Source: three-view drawing plus pictorial views. Frame: mm from the lowest corner of the part. Round coordinates to 2 decimals unless told otherwise and drop trailing zeros. Order: outer loops, then holes, each group sorted by start corner. A loop starts at its lowest first (then second) coordinate and runs counter-clockwise, first axis right, second up. Notation, with made-up numbers: (4, 81.25) -> (58, 81.25) arc R14 cw to (58, 100.25) -> close; hole circle Ø6 at (64.25, 50.25). An arc over 180 degrees is marked (long way). Answer as CSV lines item,"result". Start each with the question number.
1) Section query B-B, the plane y = 10.25. Output: boundary loops of the cut face in (x, z) (3 decimals), and give its area (3 significant figures).
2) Section query D-D, the plane z = 177.5. Output: boundary loops of the cut face in (x, y).
3) Section query A-A, the plane x = 150. Output: boundary loops of the cut face in (y, z), and give its area (3 significant figures).
4) First-contact query: P1, Ø10, axis at x = 40.5, y = 7, coming from the -Z side; P2, Ø5.5, axis at y = 5.5, z = 276, coming from the -X side; P3, Ø4, axis at y = 10.5, z = 310.5, coming from the +X side. Flat tips, straight axial feed; report the tip coordinate or a pass-through.
5) Section query C-C, the plane z = 68.5. Output: boundary loops of the cut face in (x, y).
6) Line query: L1, parallel to X at y = 4.25, z = 31.5; L2, parallel to X at y = 13.25, z = 164; L3, parallel to Z at x = 156, y = 15.75. Output: solid intervals per line, ascending.
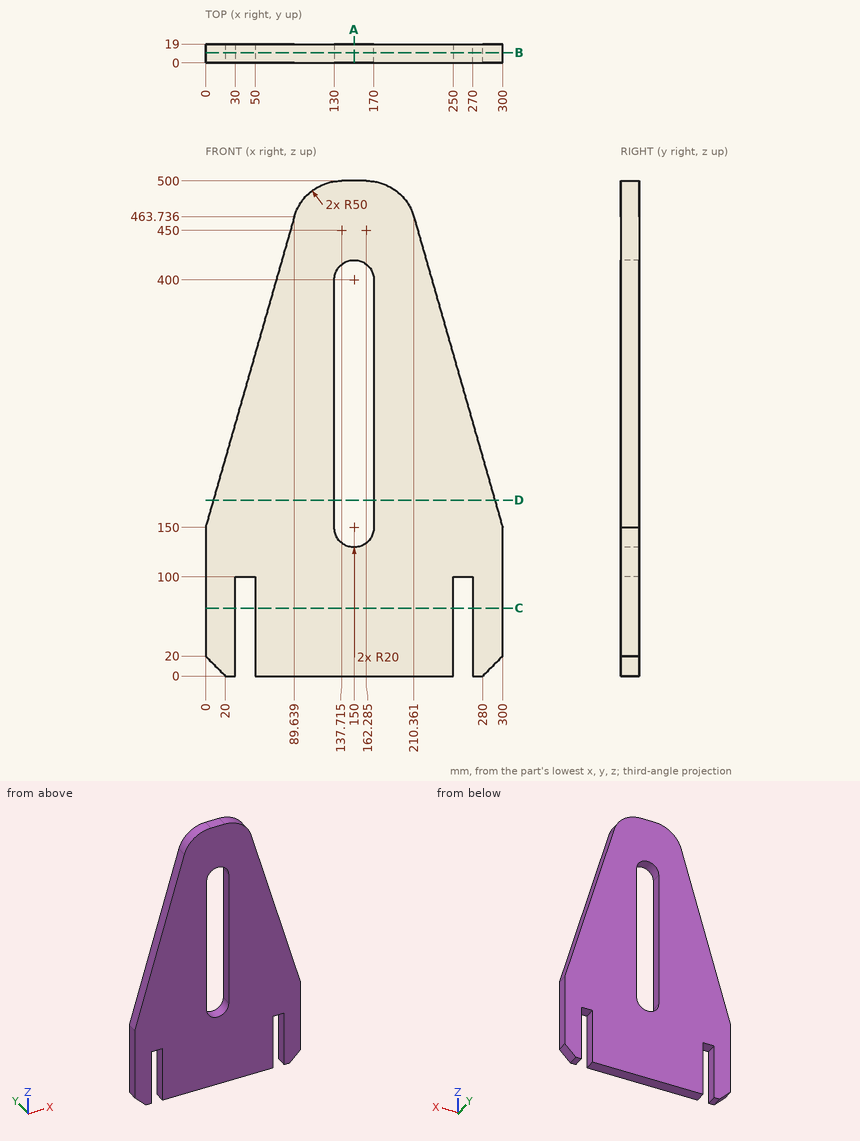
Findings:
1,outline,"(0, 20) -> (20, 0) -> (30, 0) -> (30, 100) -> (50, 100) -> (50, 0) -> (250, 0) -> (250, 100) -> (270, 100) -> (270, 0) -> (280, 0) -> (300, 20) -> (300, 150) -> (210.361, 463.736) arc R50 ccw to (162.285, 500) -> (137.715, 500) arc R50 ccw to (89.639, 463.736) -> (0, 150) -> close; hole (130, 150) arc R20 ccw to (170, 150) -> (170, 400) arc R20 ccw to (130, 400) -> close"
1,area,"98,800 mm^2"
2,outline,"(7.86, 0) -> (130, 0) -> (130, 19) -> (7.86, 19) -> close; (170, 0) -> (292.14, 0) -> (292.14, 19) -> (170, 19) -> close"
3,outline,"(0, 0) -> (19, 0) -> (19, 130) -> (0, 130) -> close; (0, 420) -> (19, 420) -> (19, 500) -> (0, 500) -> close"
3,area,"3,990 mm^2"
4,P1,"stops at z = 100"
4,P2,"stops at x = 35.21"
4,P3,"stops at x = 254.71"
5,outline,"(0, 0) -> (30, 0) -> (30, 19) -> (0, 19) -> close; (50, 0) -> (250, 0) -> (250, 19) -> (50, 19) -> close; (270, 0) -> (300, 0) -> (300, 19) -> (270, 19) -> close"
6,L1,"x = 0 to 30, 50 to 250, 270 to 300"
6,L2,"x = 4 to 130, 170 to 296"
6,L3,"z = 0 to 130.92, 419.08 to 500"
